Input: part model. Units: mm. Frame: model coordinates. Face numbers are marked on the shaded views. A direction names the side the tool comes from. Coordinates: 2 decimals unless noted, no trailing zeros. Loops run counter-clockwise (first coordinate to the right, second up) from the corner with the lowest first, then second, coordinate; pieces in that order, holes last.
Item 1: Contact query for a flat-ended pin moving along its axis: P1, Ø10, axis at y = -63.5, z = 71, coming from the -X side. Output: stop coordinate, or through.
Item 2: Section C-C on x = -69. Return loops of the section in (y, z).
Item 3: Section A-A on z = 7.2. Return loops of the section in (x, y).
Item 4: Ray query, line 1 along Y through (x, z) = (2.85, 37.5); line 2 along X through (y, z) = (27.15, 162.8); line 3 along Y through (x, z) = (3.2, 37.5). Return the intervals inside material, ascending.
Item 5: Section B-B on z = 103.5. Return loops of the section in (x, y).
Item 6: Reachability of the marked faces 1 and 2 from +Z, -Z, +X, -X, +Y, -Y: full face, straight path, thin tool, end or side. Return the list, or none.
Item 7: Section D-D on y = -1. Return loops of the section in (x, z), and give its area (3 significant figures).
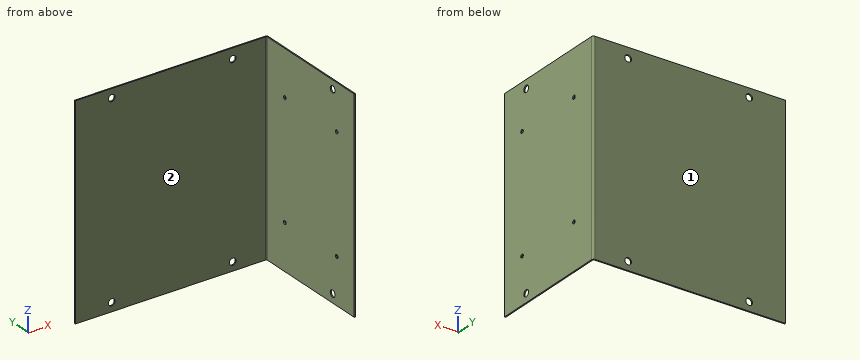
```python
from build123d import *

# Parameters (mm, degrees)
SM_BASE_FLANGE_1_DEPTH = 170
SKETCH_6_R             = 2.75
CUT_EXTRUDE_1_DEPTH    = 10
SKETCH_8_R             = 2.75
CUT_EXTRUDE_2_DEPTH    = 10
HOLE_WIZARD_3_0_3_1_D  = 3


# Sheet-metal steps are written as plain solids
with BuildPart() as part:
    # Sketch 1 → 基体-法兰1 (new body)
    with BuildSketch(Plane.XY):
        with BuildLine():
            Line((-155.610979595, 26.743544458), (1.715820405, 26.743544458))
            ThreePointArc((1.715820405, 26.743544458), (2.23667526, 26.527799313), (2.452420405, 26.006944458))
            Line((2.452420405, 26.006944458), (2.452420405, -74.456455542))
            Line((2.452420405, -74.456455542), (3.452420405, -74.456455542))
            Line((3.452420405, -74.456455542), (3.452420405, 26.006944458))
            ThreePointArc((3.452420405, 26.006944458), (2.943782042, 27.234906094), (1.715820405, 27.743544458))
            Line((1.715820405, 27.743544458), (-155.610979595, 27.743544458))
            Line((-155.610979595, 27.743544458), (-155.610979595, 26.743544458))
        make_face()
    extrude(amount=SM_BASE_FLANGE_1_DEPTH)

    # 草图6 → 切除-拉伸1 (cut)
    with BuildSketch(Plane(origin=(0, 27.743544458, 0), x_dir=(-1, 0, 0), z_dir=(0, 1, 0))):
        with Locations((125.610979595, 162.8)):
            Circle(SKETCH_6_R)
        with Locations((25.610979595, 161.523456844)):
            Circle(SKETCH_6_R)
        with Locations((25.610979595, 7.2)):
            Circle(SKETCH_6_R)
        with Locations((125.610979595, 7.2)):
            Circle(SKETCH_6_R)
    extrude(amount=-CUT_EXTRUDE_1_DEPTH, mode=Mode.SUBTRACT)

    # 草图8 → 切除-拉伸2 (cut)
    with BuildSketch(Plane(origin=(3.452420405, 0, 0), x_dir=(0, 0, -1), z_dir=(1, 0, 0))):
        with Locations(Location((-162.8, -49.456455542, 0), (0, 0, 90))):
            Circle(SKETCH_8_R)
        with Locations(Location((-7.2, -49.456455542, 0), (0, 0, 90))):
            Circle(SKETCH_8_R)
    extrude(amount=-CUT_EXTRUDE_2_DEPTH, mode=Mode.SUBTRACT)

    # Ø3.0 (3) 直径孔1 (through all)
    with Locations(Plane(origin=(3.452420405, 0, 0), x_dir=(0, 0, -1), z_dir=(1, 0, 0))):
        with Locations((-132.5, 5.757044458), (-37.5, 5.757044458), (-37.5, -54.242955542), (-132.5, -54.242955542)):
            Hole(HOLE_WIZARD_3_0_3_1_D / 2)


solid = part.part
```
Results found:
1. P1: stops at x = 2.45
2. outline: (26.74, 0) - (27.74, 0) - (27.74, 170) - (26.74, 170) - close
3. outline: (-155.61, 26.74) - (-128.36, 26.74) - (-128.36, 27.74) - (-155.61, 27.74) - close; (-122.86, 26.74) - (-28.36, 26.74) - (-28.36, 27.74) - (-122.86, 27.74) - close; (-22.86, 26.74) - (1.72, 26.74) arc R0.74 cw to (2.45, 26.01) - (2.45, -46.71) - (3.45, -46.71) - (3.45, 26.01) arc R1.74 ccw to (1.72, 27.74) - (-22.86, 27.74) - close; (2.45, -74.46) - (3.45, -74.46) - (3.45, -52.21) - (2.45, -52.21) - close
4. line 1: y = -74.46 to -55.74, -52.74 to 4.26, 7.26 to 27.32
4. line 2: x = -155.61 to -128.36, -122.86 to -28.05, -23.18 to 3.02
4. line 3: y = -74.46 to -55.74, -52.74 to 4.26, 7.26 to 26.91
5. outline: (-155.61, 26.74) - (1.72, 26.74) arc R0.74 cw to (2.45, 26.01) - (2.45, -74.46) - (3.45, -74.46) - (3.45, 26.01) arc R1.74 ccw to (1.72, 27.74) - (-155.61, 27.74) - close
6. face 1: +Z, -Z, +X, -X, +Y
6. face 2: +Z, -Z, -X, -Y
7. outline: (2.45, 0) - (3.45, 0) - (3.45, 170) - (2.45, 170) - close
7. area: 170 mm2
